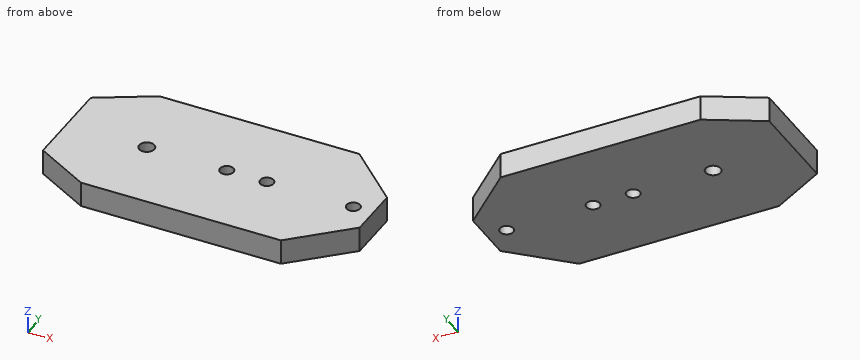
from build123d import *

# Parameters (mm, degrees)
SKETCH1_R           = 1.6
SKETCH1_R_2         = 1.8
BOSS_EXTRUDE1_DEPTH = 6


with BuildPart() as part:
    # Sketch1 → Boss-Extrude1 (new body)
    with BuildSketch(Plane.XY):
        Polygon((-19.05, -11.1), (-6.35, -18.25), (41.3, -18.25), (53.975, -6.35), (53.975, 6.35), (41.3, 18.25), (-6.35, 18.25), (-19.05, 11.1), align=None)
        with Locations((19.05, 0)):
            Circle(SKETCH1_R, mode=Mode.SUBTRACT)
        with Locations((28.6, 0)):
            Circle(SKETCH1_R, mode=Mode.SUBTRACT)
        with Locations((49.2, 0)):
            Circle(SKETCH1_R, mode=Mode.SUBTRACT)
        Circle(SKETCH1_R_2, mode=Mode.SUBTRACT)
    extrude(amount=BOSS_EXTRUDE1_DEPTH)


solid = part.part
Verification items for the finished model (mm, model axes). Round coordinates to 2 decimals unless told otherwise and drop trailing zeros. Loops run counter-clockwise (first coordinate to the right, second up) from the corner with the lowest first, then second, coordinate; pieces in that order, holes last. Notation, with made-up numbers: (48.5, 44) - (53.5, 44) arc R27 ccw to (53.5, 67) - close; hole circle Ø10 at (-10, 1.5). An arc over 180 degrees is marked (long way). Write item = value, one per line.
Q1. Sectioned sample at A-A on y = 0. Record the boundary of the cut face in (x, z) (3 decimals), plus the area to 3 significant figures.
Here are the results:
outline = (-19.05, 0) - (-1.8, 0) - (-1.8, 6) - (-19.05, 6) - close; (1.8, 0) - (17.45, 0) - (17.45, 6) - (1.8, 6) - close; (20.65, 0) - (27, 0) - (27, 6) - (20.65, 6) - close; (30.2, 0) - (47.6, 0) - (47.6, 6) - (30.2, 6) - close; (50.8, 0) - (53.975, 0) - (53.975, 6) - (50.8, 6) - close
area = 359 mm^2
Q2. Sectioned sample at B-B on x = 28.6. Record the boundary of the cut face in (y, z), plus the area to 3 significant figures.
Here are the results:
outline = (-18.25, 0) - (-1.6, 0) - (-1.6, 6) - (-18.25, 6) - close; (1.6, 0) - (18.25, 0) - (18.25, 6) - (1.6, 6) - close
area = 200 mm^2
Q3. Material ranges on L1, parallel to Y at x = 19.05, z = 1.3; L2, parallel to Y at x = 49.2, z = 2.4; L3, parallel to X at y = -13, z = 2.75, recorded low to high.
Here are the results:
L1 = -18.25 to -1.6, 1.6 to 18.25
L2 = -10.83 to -1.6, 1.6 to 10.83
L3 = -15.68 to 46.89
Q4. Sectioned sample at C-C on z = 2.5. Record the boundary of the cut face in (x, y) (3 decimals), plus the area to 3 significant figures.
Here are the results:
outline = (-19.05, -11.1) - (-6.35, -18.25) - (41.3, -18.25) - (53.975, -6.35) - (53.975, 6.35) - (41.3, 18.25) - (-6.35, 18.25) - (-19.05, 11.1) - close; hole circle Ø3.6 at (0, 0); hole circle Ø3.2 at (19.05, 0); hole circle Ø3.2 at (28.6, 0); hole circle Ø3.2 at (49.2, 0)
area = 2,390 mm^2
Q5. Sectioned sample at D-D on x = 49.2. Record the boundary of the cut face in (y, z), plus the area to 3 significant figures.
Here are the results:
outline = (-10.83, 0) - (-1.6, 0) - (-1.6, 6) - (-10.83, 6) - close; (1.6, 0) - (10.83, 0) - (10.83, 6) - (1.6, 6) - close
area = 111 mm^2
Q6. Depth check by flat-ended pin: pin 1 (2.5 mm diameter, centred on x = 19.05, y = 0, fed in from -Z). Enter the tip coordinate at first touch or a pass-through.
Here are the results:
pin_1 = through
